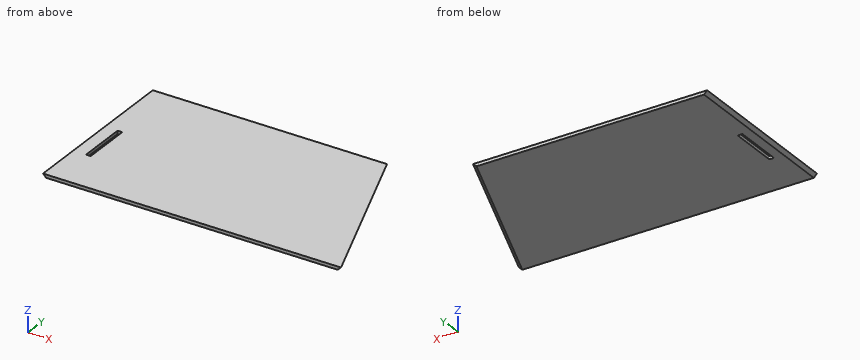
```python
from build123d import *

# Parameters (mm, degrees)
F1_DEPTH = 15
F2_SIZE  = 14.99999
F3_SIZE  = 14.99999


# Not quite as in the source:
# - a fillet or chamfer is up to 0.001 mm smaller than in the source, because OpenCascade refuses the exact size


with BuildPart() as f1:
    # F0 (on Top) → F1 (new body)
    with BuildSketch(Plane.XY):
        Polygon((0, -800), (-300, 0), (-1400, 0), (-1400, -800), align=None)
        with BuildLine():
            Line((-1340, -575), (-1340, -350))
            Line((-1340, -350), (-1318, -350))
            Line((-1318, -350), (-1318, -575))
            ThreePointArc((-1318, -575), (-1319.4644660941, -578.5355339059), (-1323, -580))
            Line((-1323, -580), (-1335, -580))
            ThreePointArc((-1335, -580), (-1338.5355339059, -578.5355339059), (-1340, -575))
        make_face(mode=Mode.SUBTRACT)
    extrude(amount=F1_DEPTH)

    # F2 (size 15 in the source; OpenCascade refuses exactly that, so slightly less here)
    f2_edges = [f1.edges().sort_by_distance(p)[0] for p in [
        (-1400, -400, 0),
    ]]
    chamfer(f2_edges, length=F2_SIZE)

    # F3 (size 15 in the source; OpenCascade refuses exactly that, so slightly less here)
    f3_edges = [f1.edges().sort_by_distance(p)[0] for p in [
        (-150, -400, 0),
    ]]
    chamfer(f3_edges, length=F3_SIZE)


solid = f1.part
```
Geometry: final body of the model. Coordinates: model frame, mm. Give positions to 0.01 mm unless a question says otherwise; leave off trailing zeros. Order: outer loops, then holes, each group sorted by start corner. A loop starts at its lowest first (then second) coordinate and runs counter-clockwise, first axis right, second up. Notation, with made-up numbers: (-33.5, 70.25) -> (-26.5, 70.25) arc R20 ccw to (-26.5, 79.25) -> close; hole circle Ø2 at (-20.5, -34.75). An arc over 180 degrees is marked (long way). Write each question's results on one line, items separated by ' | '. Start each with the question number.
1) Line query: line 1 (X direction, y = -518, z = 2.75); line 2 (X direction, y = -614, z = 6); line 3 (Z direction, x = -232, y = -213.5). Output: solid intervals per line, ascending. Write a range as from..to.
2) Section A-A (z = 2.5). Return loops of the section in (x, y), then the cut area to 3 significant figures.
3) First-contact query: pin 1 (7.5 mm diameter, centred on y = -432.5, z = 10.5, fed in from +X); pin 2 (7.5 mm diameter, centred on y = -413, z = 7, fed in from -X). Flat tips, straight axial feed; report the tip coordinate or a pass-through.
Calculated:
1) line 1: -1387.75..-1340, -1318..-118.83 | line 2: -1391..-79.36 | line 3: 3.71..15
2) outline: (-1387.5, -800) -> (-13.35, -800) -> (-313.35, 0) -> (-1387.5, 0) -> close; hole (-1340, -575) arc R5 ccw to (-1335, -580) -> (-1323, -580) arc R5 ccw to (-1318, -575) -> (-1318, -350) -> (-1340, -350) -> close | area: 974,000 mm2
3) pin 1: x = -138.37 | pin 2: x = -1395.75
